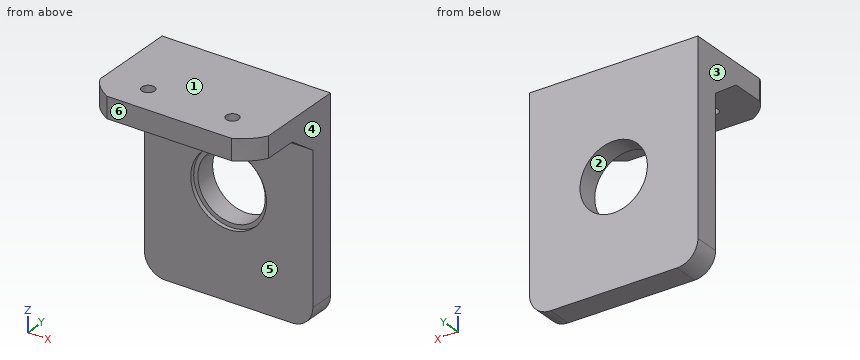
```python
from build123d import *

# Parameters (mm, degrees)
SKETCH1_W           = 40
SKETCH1_H           = 50
BOSS_EXTRUDE1_DEPTH = 6
SKETCH3_R           = 8
CUT_EXTRUDE1_DEPTH  = 9
SKETCH4_W           = 40
SKETCH4_H           = 5
BOSS_EXTRUDE2_DEPTH = 20
BOSS_EXTRUDE3_DEPTH = 40
SKETCH6_R           = 1.5
CUT_EXTRUDE2_DEPTH  = 54.150729064
CUT_EXTRUDE3_DEPTH  = 42.243181255
CUT_EXTRUDE4_DEPTH  = 54.150729064
SKETCH9_R           = 9
CUT_EXTRUDE5_DEPTH  = 1


with BuildPart() as part:
    # Sketch1 → Boss-Extrude1 (new body)
    with BuildSketch(Plane(origin=(0, 0, 0), x_dir=(1, 0, 0), z_dir=(0, 1, 0))):
        Rectangle(SKETCH1_W, SKETCH1_H)
    extrude(amount=BOSS_EXTRUDE1_DEPTH)

    # Sketch3 → Cut-Extrude1 (cut)
    with BuildSketch(Plane(origin=(0, 6, 0), x_dir=(1, 0, 0), z_dir=(0, 1, 0))):
        with Locations(Location((0, 0, 0), (0, 0, 270))):
            Circle(SKETCH3_R)
    extrude(amount=-CUT_EXTRUDE1_DEPTH, mode=Mode.SUBTRACT)

    # Sketch4 → Boss-Extrude2 (add)
    with BuildSketch(Plane.XZ):
        with Locations((0, 22.5)):
            Rectangle(SKETCH4_W, SKETCH4_H)
    extrude(amount=BOSS_EXTRUDE2_DEPTH)

    # Sketch5 → Boss-Extrude3 (add)
    with BuildSketch(Plane(origin=(20, 0, 0), x_dir=(0, 0, -1), z_dir=(1, 0, 0))):
        Polygon((-15, 0), (-20, 0), (-20, -7), align=None)
    extrude(amount=-BOSS_EXTRUDE3_DEPTH)

    # Sketch6 → Cut-Extrude2 (cut, through all)
    with BuildSketch(Plane(origin=(0, 0, 20), x_dir=(-1, 0, 0), z_dir=(0, 0, -1))):
        with Locations((-10, -13)):
            Circle(SKETCH6_R)
        with Locations((10, -13)):
            Circle(SKETCH6_R)
    extrude(amount=-CUT_EXTRUDE2_DEPTH, mode=Mode.SUBTRACT)

    # Sketch7 → Cut-Extrude3 (cut, through all)
    with BuildSketch(Plane(origin=(0, 6, 0), x_dir=(1, 0, 0), z_dir=(0, 1, 0))):
        with BuildLine():
            Line((-20, 20), (-20, 25))
            Line((-20, 25), (-15, 25))
            ThreePointArc((-15, 25), (-18.535533906, 23.535533906), (-20, 20))
        make_face()
        with BuildLine():
            Line((15, 25), (20, 25))
            Line((20, 25), (20, 20))
            ThreePointArc((20, 20), (18.535533906, 23.535533906), (15, 25))
        make_face()
    extrude(amount=-CUT_EXTRUDE3_DEPTH, mode=Mode.SUBTRACT)

    # Sketch8 → Cut-Extrude4 (cut, through all)
    with BuildSketch(Plane(origin=(0, 0, 20), x_dir=(-1, 0, 0), z_dir=(0, 0, -1))):
        with BuildLine():
            Line((20, -20), (20, -15))
            add(Edge.make_bspline(
                [(20, -15), (19.102747752, -17.059066779), (17.286957895, -18.725733446), (14.898686187, -20)],
                knots=[0, 0, 0, 0, 0.190571824, 0.190571824, 0.190571824, 0.190571824], degree=3))
            Line((14.898686187, -20), (20, -20))
        make_face()
        with BuildLine():
            Line((-20, -20), (-14.628627564, -20))
            add(Edge.make_bspline(
                [(-14.628627564, -20), (-17.085724607, -18.725733446), (-18.991534004, -17.059066779), (-20, -15)],
                knots=[0.809428176, 0.809428176, 0.809428176, 0.809428176, 1, 1, 1, 1], degree=3))
            Line((-20, -15), (-20, -20))
        make_face()
    extrude(amount=-CUT_EXTRUDE4_DEPTH, mode=Mode.SUBTRACT)

    # Sketch9 → Cut-Extrude5 (cut)
    with BuildSketch(Plane.XZ):
        with Locations(Location((0, 0, 0), (0, 0, 270))):
            Circle(SKETCH9_R)
    extrude(amount=-CUT_EXTRUDE5_DEPTH, mode=Mode.SUBTRACT)


solid = part.part
```
Model file for the job. Use its own axes, mm. Face numbers are marked on the shaded views. A direction names the side the tool comes from. Give positions to 0.01 mm unless a question says otherwise; leave off trailing zeros. Write each loop counter-clockwise with the first axis right and the second up, starting at its lowest first coordinate (ties: lowest second). Pieces come first, ordered by that corner, then holes. Notation, with made-up numbers: (37.5, 33.25) - (75.5, 33.25) arc R11 cw to (75.5, 40.25) - close; hole circle Ø4 at (84, -39.75). An arc over 180 degrees is marked (long way). One line per question, with ' | ' between items. Start each with the question number.
(1) Slice it at B-B on y = -13. Write the cut outline in (x, z), plus the area to 3 significant figures.
(2) Pin check, flat tips, straight feed: P1, Ø3, axis at x = -14.5, z = -17, coming from the -Y side; P2, Ø1, axis at x = -6, y = -8, coming from the -Z side; P3, Ø9.5, axis at x = 0, z = 0, coming from the -Y side; P4, Ø8, axis at x = -4.5, z = -4.5, coming from the +Y side. Stop position of each tip, or through.
(3) Slice it at A-A on x = 0. Write the cut outline in (y, z), plus the area to 4 significant figures.
(4) Slice it at C-C on z = 6.5. Write the cut outline in (x, y).
(5) Two-plate mould, pull along X, no slides. Class the marked faces 1, 2, 3 and 4: +X half, -X half, draft (parallel to the pull), parting line (faces both ways), or undercut.
(6) Slice it at D-D on x = -10. Write the cut outline in (y, z).
(7) 3-axis set-ups, long thin cutter, end or side, ignore diameter. For the marked faces 5 and 6: which of +Z, -Z, +X, -X, +Y, -Y reach the whole face in a straight line?
(8) Wall check: line 1 along X through (y, z) = (0.8, 0); line 2 along Y through (x, z) = (-10, 22.7); line 3 along Z through (x, y) = (-17, -7.5). Give the ranges that are in metal, low to high. Write a range as from..to.
Results below:
1) outline: (-20, 20) - (-11.5, 20) - (-11.5, 25) - (-20, 25) - close; (-8.5, 20) - (8.5, 20) - (8.5, 25) - (-8.5, 25) - close; (11.5, 20) - (20, 20) - (20, 25) - (11.5, 25) - close | area: 170 mm^2
2) P1: y = 0 | P2: z = 20 | P3: through | P4: y = 6
3) outline: (-20, 20) - (-7, 20) - (0, 15) - (0, 9) - (1, 9) - (1, 8) - (6, 8) - (6, 25) - (-20, 25) - close; (0, -25) - (6, -25) - (6, -8) - (1, -8) - (1, -9) - (0, -9) - close | area: 319.5 mm^2
4) outline: (-20, 0) - (-6.22, 0) - (-6.22, 1) - (-4.66, 1) - (-4.66, 6) - (-20, 6) - close; (4.66, 1) - (6.22, 1) - (6.22, 0) - (20, 0) - (20, 6) - (4.66, 6) - close
5) face 1: draft | face 2: undercut | face 3: -X half | face 4: +X half
6) outline: (-20, 20) - (-14.5, 20) - (-14.5, 25) - (-20, 25) - close; (-11.5, 20) - (-7, 20) - (0, 15) - (0, -25) - (6, -25) - (6, 25) - (-11.5, 25) - close
7) face 5: -Z, +X, -X, -Y | face 6: +Z, -Z, +X, -X, -Y
8) line 1: -20..-9, 9..20 | line 2: -20..-14.5, -11.5..6 | line 3: 20..25
